from build123d import *

# Parameters (mm, degrees)
SKETCH1_W            = 235
SKETCH1_H            = 235
SKETCH1_W_2          = 230
SKETCH1_H_2          = 230
EXTRUDE_THIN1_DEPTH  = 230
BOSS_EXTRUDE1_DEPTH  = 2.5
BOSS_EXTRUDE2_DEPTH  = 2.5
BOSS_EXTRUDE5_DEPTH  = 4
SKETCH8_W            = 2
SKETCH8_H            = 236.907154809
BOSS_EXTRUDE6_DEPTH  = 2
BOSS_EXTRUDE7_DEPTH  = 4
SKETCH10_W           = 2
SKETCH10_H           = 236.90715481
BOSS_EXTRUDE8_DEPTH  = 2
SKETCH11_W           = 2
SKETCH11_H           = 2
BOSS_EXTRUDE9_DEPTH  = 2
SKETCH12_W           = 2
SKETCH12_H           = 2
BOSS_EXTRUDE10_DEPTH = 2
BOSS_EXTRUDE11_DEPTH = 2


with BuildPart() as part:
    # Sketch1 → Extrude-Thin1 (new body)
    with BuildSketch(Plane(origin=(0, 0, 0), x_dir=(1, 0, 0), z_dir=(0, 1, 0))):
        with Locations((115, 115)):
            Rectangle(SKETCH1_W, SKETCH1_H)
        with Locations((115, 115)):
            Rectangle(SKETCH1_W_2, SKETCH1_H_2, mode=Mode.SUBTRACT)
    extrude(amount=EXTRUDE_THIN1_DEPTH)

    # Sketch4 → Boss-Extrude1 (add)
    with BuildSketch(Plane(origin=(232.5, 0, 0), x_dir=(0, 0, -1), z_dir=(1, 0, 0))):
        Polygon((-2.5, 230), (-2.5, 260), (232.5, 230), align=None)
    extrude(amount=-BOSS_EXTRUDE1_DEPTH)

    # Sketch5 → Boss-Extrude2 (add)
    with BuildSketch(Plane.ZY.offset(2.5)):
        Polygon((-232.5, 230), (2.5, 230), (2.5, 260), align=None)
    extrude(amount=-BOSS_EXTRUDE2_DEPTH)

    # Sketch6 → Boss-Extrude5 (add)
    with BuildSketch(Plane.ZY.offset(2.5)):
        Polygon((-232.5, 230), (2.5, 260), (2.5, 257.5), (-232.5, 227.5), align=None)
    extrude(amount=BOSS_EXTRUDE5_DEPTH)

    # Sketch8 → Boss-Extrude6 (add)
    with BuildSketch(Plane(origin=(0, 253.056792873, -32.305122494), x_dir=(1, 0, 0), z_dir=(0, -0.9919497796038491, 0.12663188675793835))):
        with Locations((-5.5, -83.365992116)):
            Rectangle(SKETCH8_W, SKETCH8_H)
    extrude(amount=BOSS_EXTRUDE6_DEPTH)

    # Sketch9 → Boss-Extrude7 (add)
    with BuildSketch(Plane(origin=(232.5, 0, 0), x_dir=(0, 0, -1), z_dir=(1, 0, 0))):
        Polygon((-2.5, 260), (232.5, 230), (232.5, 228), (-2.5, 258), align=None)
    extrude(amount=BOSS_EXTRUDE7_DEPTH)

    # Sketch10 → Boss-Extrude8 (add)
    with BuildSketch(Plane(origin=(0, 253.548775056, -32.367928731), x_dir=(1, 0, 0), z_dir=(0, -0.9919497796038491, 0.12663188675793827))):
        with Locations((235.5, -83.302676172)):
            Rectangle(SKETCH10_W, SKETCH10_H)
    extrude(amount=BOSS_EXTRUDE8_DEPTH)

    # Sketch11 → Boss-Extrude9 (add)
    with BuildSketch(Plane(origin=(0, 253.548775056, -32.367928731), x_dir=(1, 0, 0), z_dir=(0, -0.9919497796038491, 0.12663188675793827))):
        with Locations((233.5, -200.756253577)):
            Rectangle(SKETCH11_W, SKETCH11_H)
    extrude(amount=BOSS_EXTRUDE9_DEPTH)

    # Sketch12 → Boss-Extrude10 (add)
    with BuildSketch(Plane(origin=(0, 253.056792873, -32.305122494), x_dir=(1, 0, 0), z_dir=(0, -0.9919497796038491, 0.12663188675793835))):
        with Locations((-3.5, -200.81956952)):
            Rectangle(SKETCH12_W, SKETCH12_H)
    extrude(amount=BOSS_EXTRUDE10_DEPTH)

    # Sketch13 → Boss-Extrude11 (add)
    with BuildSketch(Plane.XZ):
        Polygon((-2.5, 2.5), (40.5, 2.5), (40.5, -4.341126342), (45.5, -4.341126342), (45.5, 2.5), (88.5, 2.5), (88.5, -4.341126342), (93.5, -4.341126342), (93.5, 2.5), (136.5, 2.5), (136.5, -4.341126342), (141.5, -4.341126342), (141.5, 2.5), (184.5, 2.5), (184.5, -4.341126342), (189.5, -4.341126342), (189.5, 2.5), (232.5, 2.5), (232.5, -40.5), (225.658873658, -40.5), (225.658873658, -45.5), (232.5, -45.5), (232.5, -88.5), (225.658873658, -88.5), (225.658873658, -93.5), (232.5, -93.5), (232.5, -136.5), (225.658873658, -136.5), (225.658873658, -141.5), (232.5, -141.5), (232.5, -184.5), (225.658873658, -184.5), (225.658873658, -189.5), (232.5, -189.5), (232.5, -232.5), (189.5, -232.5), (189.5, -225.658873658), (184.5, -225.658873658), (184.5, -232.5), (141.5, -232.5), (141.5, -225.658873658), (136.5, -225.658873658), (136.5, -232.5), (93.5, -232.5), (93.5, -225.658873658), (88.5, -225.658873658), (88.5, -232.5), (45.5, -232.5), (45.5, -225.658873658), (40.5, -225.658873658), (40.5, -232.5), (-2.5, -232.5), (-2.5, -189.5), (4.341126342, -189.5), (4.341126342, -184.5), (-2.5, -184.5), (-2.5, -141.5), (4.341126342, -141.5), (4.341126342, -136.5), (-2.5, -136.5), (-2.5, -93.5), (4.341126342, -93.5), (4.341126342, -88.5), (-2.5, -88.5), (-2.5, -45.5), (4.341126342, -45.5), (4.341126342, -40.5), (-2.5, -40.5), align=None)
    extrude(amount=BOSS_EXTRUDE11_DEPTH)


solid = part.part
Here's how the part is built. I have some questions about the finished solid (model axes, mm). A direction names the side the tool comes from. Coordinates: 2 decimals unless noted, no trailing zeros. Order: outer loops, then holes, each group sorted by start corner. A loop starts at its lowest first (then second) coordinate and runs counter-clockwise, first axis right, second up. Notation, with made-up numbers: M 74.5,23 L 105.5,23 A22 cw 105.5,41 Z; hole C 38,61 d10. An arc over 180 degrees is marked long. Answer as CSV lines item,"result". Start each with the question number.
1. I need wall thicknesses on line 1 (X direction, y = 81.5, z = -13); line 2 (Z direction, x = 181, y = 61.5); line 3 (Y direction, x = 115.5, z = -192). Which ranges of each line are inside material? Lowest first, please. Write a range as [from, to].
2. For pin 1 (2 mm diameter, centred on x = 196.5, z = -128.5, fed in from +Y); pin 2 (3 mm diameter, centred on x = 91.5, z = 1.5, fed in from -Y); pin 3 (1 mm diameter, centred on y = -1, z = -186, fed in from -X), each with a flat end and sliding along its axis, tell me the tip position at first contact or that it passes through.
3. We'd pull the mould along Z, two halves only. Please class faces 1 (the flat face through (113, 113, 0)), 2 (the flat face through (236.5, 243, -117)), 3 (the flat face through (233.2, 245.21, -113.36)): released by +Z, released by -Z, zero draft, split by the parting line, or undercut.
4. On a 3-axis mill with a long thin cutter (end or side, diameter ignored), from which of +Z, -Z, +X, -X, +Y, -Y can I reach the whole of each face in a straight line? I mean faces 4 (the flat face through (0, 132, -117)), 5 (the flat face through (-5.417, 240.726, -113.102)), 6 (the flat face through (234.5, 242, -116)), 7 (the flat face through (235.805, 241.226, -113.102)), 8 (the flat face through (117, 116, -232.5)). Say none if no direction works.
5. I want a section at C-C, the plane z = -106.5. Write out the boundary of the cut face in (x, y), and give its area (3 significant figures).
6. I want a section at D-D, the plane z = -207. Write out the boundary of the cut face in (x, y).
7. I want a section at B-B, the plane x = 129.5. Write out the boundary of the cut face in (y, z), and give its area (3 significant figures).
8. I want a section at A-A, the plane y = 108. Write out the boundary of the cut face in (x, z), and give its area (4 significant figures).
Recorded:
1,line 1,"x = [-2.5, 0], [230, 232.5]"
1,line 2,"z = [-232.5, -230], [0, 2.5]"
1,line 3,"y = [-2, 0]"
2,pin 1,"stops at y = 0"
2,pin 2,"stops at y = 0"
2,pin 3,"stops at x = 4.34"
3,face 1,"undercut"
3,face 2,"zero draft"
3,face 3,"released by -Z"
4,face 4,"+Y"
4,face 5,"+Z, -X, -Y"
4,face 6,"+Z, -Y"
4,face 7,"+Z, +X, -Y"
4,face 8,"-Z, +X, -X, +Y, -Y"
5,outline,"M -6.5,241.57 L -4.5,241.57 L -4.5,243.59 L -2.5,243.59 L -2.5,-2 L 232.5,-2 L 232.5,244.09 L 234.5,244.09 L 234.5,242.07 L 236.5,242.07 L 236.5,246.09 L 230,246.09 L 230,0 L 0,0 L 0,246.09 L -6.5,246.09 Z"
5,area,"1,730 mm2"
6,outline,"M -6.5,228.74 L -4.5,228.74 L -4.5,230.76 L -2.5,230.76 L -2.5,-2 L 232.5,-2 L 232.5,231.26 L 234.5,231.26 L 234.5,229.24 L 236.5,229.24 L 236.5,233.26 L 230,233.26 L 230,0 L 0,0 L 0,233.26 L -6.5,233.26 Z"
7,outline,"M -2,-232.5 L 230,-232.5 L 230,-230 L 0,-230 L 0,0 L 230,0 L 230,2.5 L -2,2.5 Z"
7,area,"1,620 mm2"
8,outline,"M -2.5,-232.5 L 232.5,-232.5 L 232.5,2.5 L -2.5,2.5 Z; hole M 0,-230 L 230,-230 L 230,0 L 0,0 Z"
8,area,"2,325 mm2"
